```python
from build123d import *

# Parameters (mm, degrees)
SKETCH1_R           = 50.8
SKETCH1_R_2         = 25.4
SKETCH1_R_3         = 1.5875
SKETCH1_W           = 9.525
SKETCH1_H           = 3.175
SKETCH1_W_2         = 3.175
SKETCH1_H_2         = 9.525
BOSS_EXTRUDE1_DEPTH = 3.175


with BuildPart() as part:
    # Sketch1 → Boss-Extrude1 (new body)
    with BuildSketch(Plane.XY):
        with Locations((-3.17373, 0)):
            Circle(SKETCH1_R)
        with Locations((-3.17373, 0)):
            Circle(SKETCH1_R_2, mode=Mode.SUBTRACT)
        with Locations((-3.17373, -33.8709)):
            Circle(SKETCH1_R_3, mode=Mode.SUBTRACT)
        with Locations((30.69717, 0)):
            Circle(SKETCH1_R_3, mode=Mode.SUBTRACT)
        with Locations((-37.04463, 0)):
            Circle(SKETCH1_R_3, mode=Mode.SUBTRACT)
        with Locations((-3.17373, 33.8709)):
            Circle(SKETCH1_R_3, mode=Mode.SUBTRACT)
        with Locations((-37.01923, -20.6375)):
            Rectangle(SKETCH1_W, SKETCH1_H, mode=Mode.SUBTRACT)
        with Locations((-37.01923, 20.6375)):
            Rectangle(SKETCH1_W, SKETCH1_H, mode=Mode.SUBTRACT)
        with Locations((-23.81123, 33.8455)):
            Rectangle(SKETCH1_W_2, SKETCH1_H_2, mode=Mode.SUBTRACT)
        with Locations((17.46377, 33.8455)):
            Rectangle(SKETCH1_W_2, SKETCH1_H_2, mode=Mode.SUBTRACT)
        with Locations((17.46377, -33.8455)):
            Rectangle(SKETCH1_W_2, SKETCH1_H_2, mode=Mode.SUBTRACT)
        with Locations((-23.81123, -33.8455)):
            Rectangle(SKETCH1_W_2, SKETCH1_H_2, mode=Mode.SUBTRACT)
        with Locations((30.67177, -20.6375)):
            Rectangle(SKETCH1_W, SKETCH1_H, mode=Mode.SUBTRACT)
        with Locations((30.69717, 20.6375)):
            Rectangle(SKETCH1_W, SKETCH1_H, mode=Mode.SUBTRACT)
    extrude(amount=BOSS_EXTRUDE1_DEPTH)


solid = part.part
```
Geometry: final body of the model. Coordinates: model frame, mm. Round coordinates to 2 decimals unless told otherwise and drop trailing zeros. Loops run counter-clockwise (first coordinate to the right, second up) from the corner with the lowest first, then second, coordinate; pieces in that order, holes last. Notation, with made-up numbers: (84.25, -18) -> (116.25, -18) arc R18 ccw to (116.25, 8) -> close; hole circle Ø8 at (69, 60.25). An arc over 180 degrees is marked (long way). Use one line per item in the form item = value. Start each with the question number.
1) Section B-B on x = -21. Output: boundary loops of the cut face in (y, z) (3 decimals), then the cut area to 3 significant figures.
2) Line query: L1, parallel to X at y = -34, z = 0.6; L2, parallel to X at y = 21, z = 1.65; L3, parallel to Y at x = -39, z = 0.35 (3 decimals). Output: solid intervals per line, ascending.
3) First-contact query: P1, Ø1, axis at x = -23, z = 1.5, coming from the +Y side; P2, Ø1.6, axis at y = -35.5, z = 1, coming from the -X side; P3, Ø1.6, axis at x = -23.5, z = 1, coming from the -Y side. Flat tips, straight axial feed; report the tip coordinate or a pass-through.
4) Section D-D on x = 27.5. Output: boundary loops of the cut face in (y, z) (3 decimals), then the cut area to 3 significant figures.
5) Section A-A on y = 0. Output: boundary loops of the cut face in (x, z) (3 decimals).
6) Draft query along Y for faces 1 (the cylindrical face through (45.28, 15.26, 1.57)), 2 (the flat face through (-22.224, 34, 2)), 3 (the flat face through (-37, -22.225, 2)), 4 (the flat face through (-26, 12, 0)). Return one class per face: released by +Y, released by -Y, zero draft, split by the parting line, or undercut.
7) Section C-C on y = 37. Output: boundary loops of the cut face in (x, z) (3 decimals).
Response:
q1.outline = (-47.57, 0) -> (-18.094, 0) -> (-18.094, 3.175) -> (-47.57, 3.175) -> close; (18.094, 0) -> (47.57, 0) -> (47.57, 3.175) -> (18.094, 3.175) -> close
q1.area = 187 mm^2
q2.L1 = -40.92 to -25.4, -22.22 to -4.76, -1.59 to 15.88, 19.05 to 34.57
q2.L2 = -49.43 to -41.78, -32.26 to -17.46, 11.11 to 25.93, 35.46 to 43.08
q2.L3 = -36.016 to -22.225, -19.05 to 19.05, 22.225 to 36.016
q3.P1 = 46.98
q3.P2 = -40.28
q3.P3 = -46.9
q4.outline = (-40.494, 0) -> (-22.225, 0) -> (-22.225, 3.175) -> (-40.494, 3.175) -> close; (-19.05, 0) -> (19.05, 0) -> (19.05, 3.175) -> (-19.05, 3.175) -> close; (22.225, 0) -> (40.494, 0) -> (40.494, 3.175) -> (22.225, 3.175) -> close
q4.area = 237 mm^2
q5.outline = (-53.974, 0) -> (-38.632, 0) -> (-38.632, 3.175) -> (-53.974, 3.175) -> close; (-35.457, 0) -> (-28.574, 0) -> (-28.574, 3.175) -> (-35.457, 3.175) -> close; (22.226, 0) -> (29.11, 0) -> (29.11, 3.175) -> (22.226, 3.175) -> close; (32.285, 0) -> (47.626, 0) -> (47.626, 3.175) -> (32.285, 3.175) -> close
q6.face_1 = split by the parting line
q6.face_2 = undercut
q6.face_3 = undercut
q6.face_4 = zero draft
q7.outline = (-37.982, 0) -> (-25.399, 0) -> (-25.399, 3.175) -> (-37.982, 3.175) -> close; (-22.224, 0) -> (15.876, 0) -> (15.876, 3.175) -> (-22.224, 3.175) -> close; (19.051, 0) -> (31.635, 0) -> (31.635, 3.175) -> (19.051, 3.175) -> close
